Check sheet for the modelled part. Datum: model origin and axes. Units: mm. A direction names the side the tool comes from. Give positions to 0.01 mm unless a question says otherwise; leave off trailing zeros. Write each loop counter-clockwise with the first axis right and the second up, starting at its lowest first coordinate (ties: lowest second). Pieces come first, ordered by that corner, then holes. Notation, with made-up numbers: M 72,36 L 110,36 A38 cw 110,75 Z; hole C -34,53.5 d5. An arc over 180 degrees is marked long. One line per item, written item: value. Start each with the question number.
from build123d import *

# Parameters (mm, degrees)
CHAFL_N1_SIZE         = 5
CHAFL_N2_SIZE         = 5
CHAFL_N2_SIZE2        = 2.886751346
REDONDEO1_R           = 1.5
CORTAR_EXTRUIR1_DEPTH = 40
CROQUIS3_R            = 6
CORTAR_EXTRUIR2_DEPTH = 40


with BuildPart() as part:
    # Croquis1 → Revolución1 (revolve)
    with BuildSketch(Plane.XY, mode=Mode.PRIVATE) as revoluci_n1_sk:
        with BuildLine():
            Line((0, -80), (0, 80))
            ThreePointArc((0, 80), (-9.848857802, 73.599492356), (-8, 62))
            Line((-8, 62), (-8, 50))
            Line((-8, 50), (-15, 50))
            Line((-15, 50), (-15, 40))
            Line((-15, 40), (-35, 40))
            Line((-35, 40), (-35, 32))
            Line((-35, 32), (-10, 32))
            Line((-10, 32), (-10, 30))
            Line((-10, 30), (-14.5, 30))
            Line((-14.5, 30), (-14.5, 20))
            Line((-14.5, 20), (-7.5, 20))
            Line((-7.5, 20), (-7.5, -80))
            Line((-7.5, -80), (0, -80))
        make_face()
    revolve(revoluci_n1_sk.sketch.rotate(Axis((0, -80, 0), (0, 1, 0)), 180), axis=Axis((0, -80, 0), (0, 1, 0)))

    # Chaflán1
    # the kernel refuses this chamfer: 5 mm, written as the material it takes off along each edge
    with BuildSketch(Plane(origin=(0, 30, 0), x_dir=(1, 0, 0), z_dir=(0, 0, 1))) as chafl_n1_piece_1_section:
        Polygon((14.5 - CHAFL_N1_SIZE, 0), (14.5, -CHAFL_N1_SIZE), (14.5, 0), align=None)
    chafl_n1_piece_1 = revolve(axis=Axis((0, 30, 0), (0, 1, 0)), mode=Mode.PRIVATE)
    chafl_n1_piece_1 = chafl_n1_piece_1 - Plane(origin=(0, 27.252174823, 0), x_dir=(1, 0, 0), z_dir=(0, -1, 0)) * Cylinder(10, 58, mode=Mode.PRIVATE)
    add(chafl_n1_piece_1, mode=Mode.SUBTRACT)

    # Chaflán2
    chafl_n2_edges = [part.edges().sort_by_distance(p)[0] for p in [
        (-35, 40, 0),
    ]]
    chafl_n2_side = [part.faces().sort_by_distance(p)[0] for p in [
        (-15.989949494, 40, 0),
    ]]
    chamfer(chafl_n2_edges, length=CHAFL_N2_SIZE, length2=CHAFL_N2_SIZE2, reference=chafl_n2_side[0])

    # Redondeo1
    redondeo1_edges = [part.edges().sort_by_distance(p)[0] for p in [
        (-15, 50, 0),
    ]]
    fillet(redondeo1_edges, radius=REDONDEO1_R)

    # Croquis2 → Cortar-Extruir1 (cut, symmetric)
    with BuildSketch(Plane.XY):
        Polygon((-13.5, 50), (-5.5, 50), (-5.5, 83.023482793), (-17.692901936, 83.023482793), (-17.692901936, 50), align=None)
    cortar_extruir1 = extrude(amount=CORTAR_EXTRUIR1_DEPTH, both=True, mode=Mode.SUBTRACT)

    # Simetría1: Cortar-Extruir1 across plane
    add(cortar_extruir1.mirror(Plane(origin=(0, 0, 0), x_dir=(0, 0, 1), z_dir=(1, 0, 0))), mode=Mode.SUBTRACT)

    # Croquis3 → Cortar-Extruir2 (cut, symmetric)
    with BuildSketch(Plane(origin=(5.5, 0, 0), x_dir=(0, 0, -1), z_dir=(1, 0, 0))):
        with Locations(Location((0, 69.222222222, 0), (0, 0, 270))):
            Circle(CROQUIS3_R)
    extrude(amount=CORTAR_EXTRUIR2_DEPTH, both=True, mode=Mode.SUBTRACT)


solid = part.part
1) Cross-section at D-D (y = -64.5). Record the boundary of the cut face in (x, z), plus the area to 3 significant figures.
2) Cross-section at C-C (y = 70). Record the boundary of the cut face in (x, z), plus the area to 3 significant figures.
3) Draft check along Y on faces 1 (the cylindrical face through (0.08, 63.68, 2.3)), 2 (the conical face through (28.91, 39.82, -9.11)), 3 (the cylindrical face through (-7.587, 34.521, 34.168)), 4 (the cylindrical face through (0, 56, 8)). Enter one of: released by +Y, released by -Y, zero draft, split by the parting line, or undercut.
4) Gauge pin test, flat ends, axial feed: pin 1 (12 mm diameter, centred on y = 35.5, z = -14, fed in from +X); pin 2 (4 mm diameter, centred on x = 21, z = 21.5, fed in from -Y); pin 3 (12 mm diameter, centred on x = 19, z = 4.5, fed in from +Y). Record the tip position at first contact, or that the pin passes through.
5) Tool access check on faces 5 (the flat face through (6, 20, 6)), 6 (the cylindrical face through (0, 56, -8)), 7 (the flat face through (-5.5, 61, 0)), 8 (the flat face through (-6, 40, -14)). Record the directions out of +Z, -Z, +X, -X, +Y, -Y that give a thin tool (end or side, any length) a straight path to the whole face; none if there is none.
6) Material ranges on L1, parallel to Y at x = 24, z = 6; L2, parallel to X at y = 5, z = -4.5; L3, parallel to Z at x = -13, y = 41.5, recorded low to high. Write a range as from..to.
Data:
1. outline: C 0,0 d15
1. area: 177 mm2
2. outline: M -5.5,-9.24 A10.75 ccw 5.5,-9.24 L 5.5,-5.95 L -5.5,-5.95 Z; M -5.5,5.95 L 5.5,5.95 L 5.5,9.24 A10.75 ccw -5.5,9.24 Z
2. area: 94.8 mm2
3. face 1: undercut
3. face 2: released by +Y
3. face 3: zero draft
3. face 4: undercut
4. pin 1: stops at x = 34.07
4. pin 2: stops at y = 32
4. pin 3: stops at y = 50
5. face 5: -Y
5. face 6: -Z
5. face 7: +Z, -Z, -X, +Y
5. face 8: +Y
6. L1: y = 32..40
6. L2: x = -6..6
6. L3: z = -7.48..7.48
